Build history of the part. All positions in model axes, mm. A direction names the side the tool comes from. Coordinates: 2 decimals unless noted, no trailing zeros. Write each question's results on one line, items separated by ' | '. Start each with the question number.
Q1. Drop flat-ended pins along their axis: pin 1 Ø2 at (y, z) = (-133, -15) entering from -X; pin 2 Ø2 at (x, y) = (0, -49.5) entering from -Z; pin 3 Ø10 at (y, z) = (-21.5, -16.5) entering from +X; pin 4 Ø1.5 at (y, z) = (-72.5, -9) entering from -X. Give the stop position or say it passes through.
Q2. Drill centre lines: line 1 (Z direction, x = 20, y = -56); line 2 (Z direction, x = -15, y = -44.5); line 3 (X direction, y = -108.5, z = -26). Where is each one in solid material? Low to high.
Q3. Tool access for faces 1 (the face through (-0.759, -72.854, -9.511)), 2 (the face through (3.014, -0.452, -27.823)): list every direction of +Z, -Z, +X, -X, +Y, -Y with a clear straight run to the whole face (end or side of a thin tool).
from build123d import *


with BuildPart() as f6:
    # F5 (on face) → F6 section 0
    with BuildSketch(Plane(origin=(0, -2.86481, -0.250638), x_dir=(-1, 0, 0), z_dir=(0, 0.996195, 0.087156))):
        Polygon((-38.1, 32.87001), (-76.2, -32.87001), (76.2, -32.87001), (38.1, 32.87001), align=None)
    # F2 (on offset) → F6 section 1
    with BuildSketch(Plane.XZ.offset(203.2)):
        Polygon((-15.24, 0), (-27.94, -21.997045), (27.94, -21.997045), (15.24, 0), align=None)
    loft()

    # F10 (on face) → F11 section 0
    with BuildSketch(Plane(origin=(0, -65.596307, 17.576477), x_dir=(1, 0, 0), z_dir=(0, -0.965926, 0.258819))):
        Polygon((-76.2, -40.969525), (76.2, -40.969525), (60.96, -15.472508), (-60.96, -15.472508), align=None)
    # F3 (on Front) → F11 section 1
    with BuildSketch(Plane.XZ):
        Polygon((76.2, -21.997045), (57.15, 10.998523), (-57.15, 10.998523), (-76.2, -21.997045), align=None)
    loft(mode=Mode.SUBTRACT)


solid = f6.part
Returned:
1) pin 1: stops at x = -39.08 | pin 2: stops at z = -30.37 | pin 3: passes through | pin 4: stops at x = -47.91
2) line 1: z = -29.96 to -22, 4.27 to 24.22 | line 2: z = -30.59 to -22, 5.65 to 26.11 | line 3: x = -49.79 to 49.79
3) face 1: +X, -X, +Y | face 2: +Z, +X, -X, +Y
